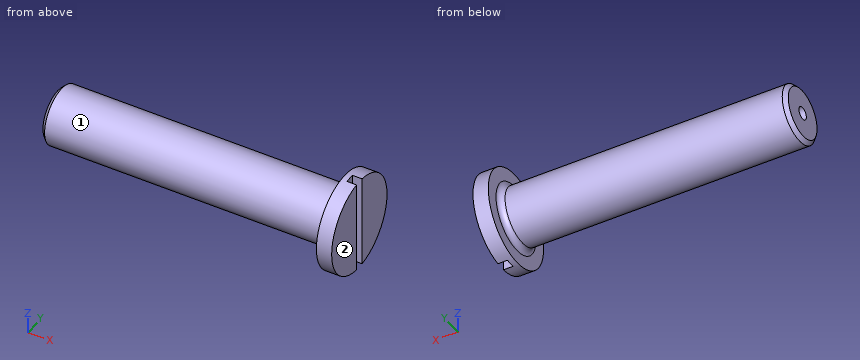
Autodesk Inventor part; units mm, degrees
ref_plane "YZ Plane" through (0, 0, 0) normal (1, 0, 0) x (0, 1, 0)
ref_plane "XZ Plane" through (0, 0, 0) normal (0, 1, 0) x (-1, 0, 0)
ref_plane "XY Plane" through (0, 0, 0) normal (0, 0, 1) x (1, 0, 0)
sketch "Sketch1" plane through (0, 0, 0) normal (0, 0, 1) x (1, 0, 0)
  line L0 (0, 0) -> (150, 0)
  line L1 (150, 0) -> (150, 15)
  line L2 (150, 15) -> (0, 15)
  line L3 (0, 15) -> (0, 0)
  line L4 (150, 0) -> (158, 0)
  line L5 (158, 0) -> (158, 25)
  line L6 (158, 25) -> (150, 25)
  line L7 (150, 25) -> (150, 0)
  dimension "d0" = 15
  dimension "d1" = 25
  dimension "d2" = 150
  dimension "d3" = 8
revolve "Revolution1" add sketch "Sketch1" angle 360 about axis through (0, 0, 0) along (1, 0, 0)
fillet "Fillet1" radius 3 1 edges at (150, -15, 0)
chamfer "Chamfer1" distance 2 angle 45 1 edges at (0, -15, 0)
sketch "Sketch2" plane through (0, 0, 0) normal (-1, 0, 0) x (0, 0, 1)
  point P0 (0, 0)
  point P1 (0, 0)
hole "Hole1" at (0, 0, 0) direction (1, 0, 0) diameter 6.647 depth 22.2 tip angle 118
sketch "Sketch3" plane through (158, 0, 0) normal (1, 0, 0) x (0, 0, -1)
  line L0 (-25, 2.5) -> (25, 2.5)
  line L1 (25, 2.5) -> (25, -2.5)
  line L2 (25, -2.5) -> (-25, -2.5)
  line L3 (-25, -2.5) -> (-25, 2.5)
  circle A0 centre (0, 0) radius 18
  circle A1 centre (0, 0) radius 25
  dimension "d16" = 50
  dimension "d17" = 50
  dimension "d18" = 25
  dimension "d19" = 5
  dimension "d20" = 2.5
extrude "Extrusion1" cut sketch "Sketch3" against normal blind 5 contours L0 A1 L3 | L0 A0 L2 A1 | A1 L2 L3 | L0 A0 L2 | A1 L2 A0 L0 | L0 L1 A1 | L1 L2 A1
equation "\"d17\" = d16"
properties part number "Top_Hinge Cylinder Long" material "Stainless Steel"
Work out the finished part from the listing and answer in its coordinate system (mm). Face numbers are marked on the shaded views. A direction names the side the tool comes from. Give positions to 0.01 mm unless a question says otherwise; leave off trailing zeros. Order: outer loops, then holes, each group sorted by start corner. A loop starts at its lowest first (then second) coordinate and runs counter-clockwise, first axis right, second up. Notation, with made-up numbers: (71, -26.75) - (97, -26.75) arc R21 ccw to (97, -4.75) - close; hole circle Ø6 at (69, 84.25). An arc over 180 degrees is marked (long way). Answer as CSV lines item,"result". Start each with the question number.
Q1. The part is cut by section A-A (x = 16). Write down the section's boundary in (y, z).
Q2. Find the intervals of material crossed by L1, parallel to Z at x = 7, y = 0; L2, parallel to X at y = -20, z = 2; L3, parallel to Z at x = 49.5, y = 0.5, in increasing order. Write a range as [from, to].
Q3. The part is cut by section C-C (x = 124). Write down the section's boundary in (y, z), then the cut area to 3 significant figures.
Q4. Given pin 1 Ø12 at (x, z) = (92, -15.5) entering from -Y; pin 2 Ø12 at (y, z) = (14, -5) entering from -X; pin 3 Ø1.5 at (x, z) = (155.5, -11) entering from -Y; pin 4 Ø10 at (y, z) = (-10, -17) entering from -X, each flat-ended and moving along its own axis, determine where each tip first touches the part or whether it passes through.
Q5. The part is cut by section B-B (z = 19.5). Write down the section's boundary in (x, y).
Q6. For the marked faces 1 and 2, determine the directions among +Z, -Z, +X, -X, +Y, -Y from which every point of the face is accessible in a straight line to the end or side of a thin tool.
Check result:
1,outline,"circle Ø30 at (0, 0); hole circle Ø6.65 at (0, 0)"
2,L1,"z = [-15, -3.32], [3.32, 15]"
2,L2,"x = [150, 158]"
2,L3,"z = [-14.99, 14.99]"
3,outline,"circle Ø30 at (0, 0)"
3,area,"707 mm²"
4,pin 1,"stops at y = -11.61"
4,pin 2,"stops at x = 0"
4,pin 3,"stops at y = -22.8"
4,pin 4,"stops at x = 1.72"
5,outline,"(150, -15.64) - (158, -15.64) - (158, -2.5) - (153, -2.5) - (153, 2.5) - (158, 2.5) - (158, 15.64) - (150, 15.64) - close"
6,face 1,"-X"
6,face 2,"+Z, -Z, +X, +Y, -Y"
